```python
from build123d import *

# Parameters (mm, degrees)
BOSS_EXTRUDE1_DEPTH     = 2.54
SKETCH2_R               = 1
CUT_EXTRUDE1_DEPTH      = 3.54
CUT_EXTRUDE1_DEPTH_BACK = 1


with BuildPart() as part:
    # Sketch1 → Boss-Extrude1 (new body)
    with BuildSketch(Plane(origin=(0, 0, 0), x_dir=(1, 0, 0), z_dir=(0, 1, 0))):
        with BuildLine():
            Line((-15, 2.5), (15, 2.5))
            ThreePointArc((15, 2.5), (17.5, 0), (15, -2.5))
            Line((15, -2.5), (-15, -2.5))
            ThreePointArc((-15, -2.5), (-17.5, 0), (-15, 2.5))
        make_face()
    extrude(amount=BOSS_EXTRUDE1_DEPTH)

    # Sketch2 → Cut-Extrude1 (cut, two sides)
    with BuildSketch(Plane(origin=(0, 0, 0), x_dir=(1, 0, 0), z_dir=(0, 1, 0))) as cut_extrude1_sk:
        with Locations((-15, 0)):
            Circle(SKETCH2_R)
        with Locations((15, 0)):
            Circle(SKETCH2_R)
    extrude(amount=CUT_EXTRUDE1_DEPTH, mode=Mode.SUBTRACT)
    extrude(cut_extrude1_sk.sketch, amount=-CUT_EXTRUDE1_DEPTH_BACK, mode=Mode.SUBTRACT)


solid = part.part
```
Input: part model. Units: mm. Frame: model coordinates. Coordinates: 2 decimals unless noted, no trailing zeros. Write each loop counter-clockwise with the first axis right and the second up, starting at its lowest first coordinate (ties: lowest second). Pieces come first, ordered by that corner, then holes. Notation, with made-up numbers: M 19.5,-34.75 L 72.5,-34.75 A19 ccw 72.5,-20.75 Z; hole C -4.75,48.5 d6. An arc over 180 degrees is marked long. Use one line per item in the form item = value.
Q1. First-contact query: pin 1 (1.6 mm diameter, centred on x = -15, z = 0, fed in from +Y); pin 2 (1 mm diameter, centred on y = 0.5, z = 1.5, fed in from +X); pin 3 (1.5 mm diameter, centred on y = 1, z = 0.5, fed in from -X). Flat tips, straight axial feed; report the tip coordinate or a pass-through.
Answer below:
pin_1 = through
pin_2 = 17.29
pin_3 = -17.5
Q2. Section B-B (y = 0.6). Return loops of the section in (x, z), plus the area to 3 significant figures.
Answer below:
outline = M -15,-2.5 L 15,-2.5 A2.5 ccw 15,2.5 L -15,2.5 A2.5 ccw Z; hole C -15,0 d2; hole C 15,0 d2
area = 163 mm²
Q3. Draft query along Z for faces 1 (the face through (0, 1, -2.5)), 2 (the face through (-14, 1, 0)), 3 (the face through (0, 1, 2.5)). Return one class per face: released by +Z, released by -Z, zero draft, split by the parting line, or undercut.
Answer below:
face_1 = released by -Z
face_2 = undercut
face_3 = released by +Z
Q4. Section A-A (z = 0). Return loops of the section in (x, y).
Answer below:
outline = M -17.5,0 L -16,0 L -16,2.54 L -17.5,2.54 Z; M -14,0 L 14,0 L 14,2.54 L -14,2.54 Z; M 16,0 L 17.5,0 L 17.5,2.54 L 16,2.54 Z
Q5. Section C-C (z = -1.55). Return loops of the section in (x, y), plus the area to 3 significant figures.
Answer below:
outline = M -16.96,0 L 16.96,0 L 16.96,2.54 L -16.96,2.54 Z
area = 86.2 mm²
Q6. Material intervals for probe 1 along X at (y, z) = (1.3, 0); probe 2 along Z at (x, y) = (-15, 1); probe 3 along X at (y, z) = (2.1, -0.6), sorted ascending. Write a range as from..to.
Answer below:
probe_1 = -17.5..-16, -14..14, 16..17.5
probe_2 = -2.5..-1, 1..2.5
probe_3 = -17.43..-15.8, -14.2..14.2, 15.8..17.43
